Part print with two shaded views. Sizes in mm from the minimum x, y, z corner. Give positions to 0.01 mm unless a question says otherwise; leave off trailing zeros. Order: outer loops, then holes, each group sorted by start corner. A loop starts at its lowest first (then second) coordinate and runs counter-clockwise, first axis right, second up.
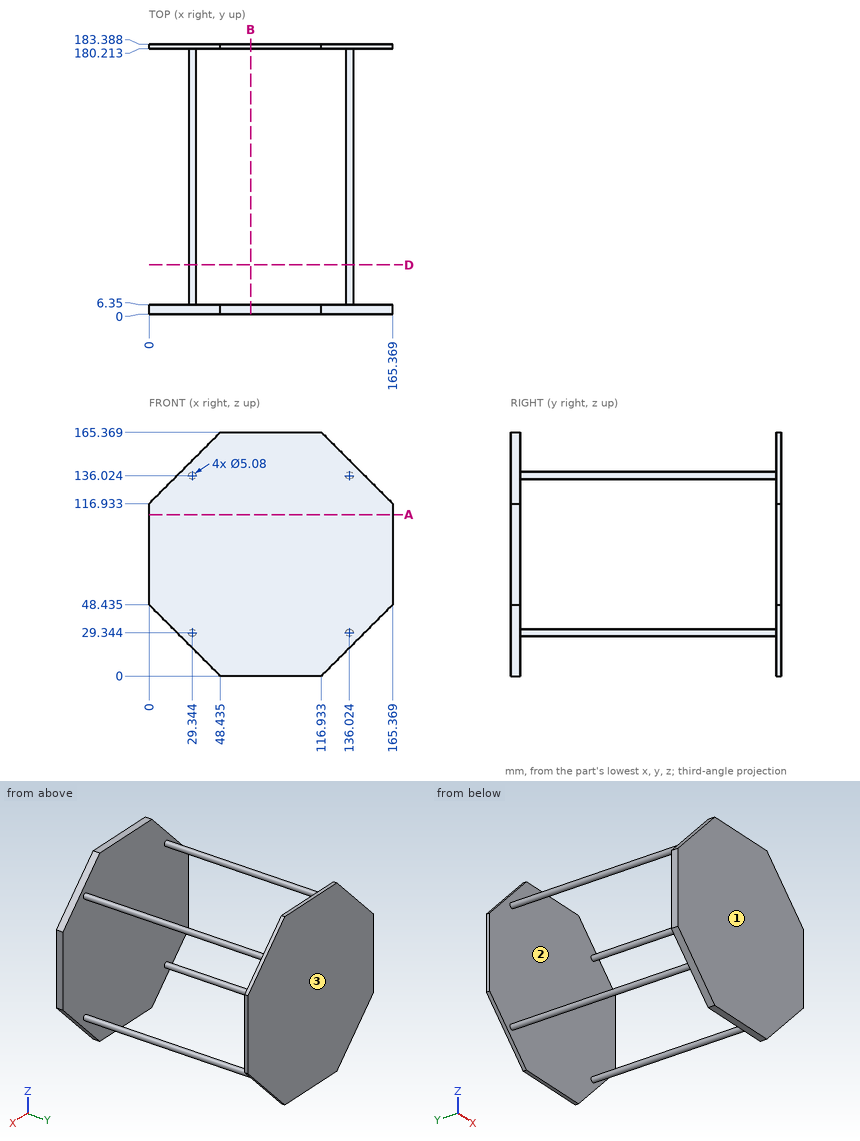
Item 1: Two-plate mould, pull along Y, no slides. Class the marked faces 1, 2 and 3: released by +Y, released by -Y, zero draft, split by the parting line, or undercut.
Item 2: Drop flat-ended pins along their axis: pin 1 Ø6 at (x, z) = (108.5, 73) entering from -Y; pin 2 Ø12 at (x, y) = (41.5, 66) entering from +Z; pin 3 Ø1.5 at (x, y) = (135, 35.5) entering from +Z. Give the stop position or say it passes through.
Item 3: Slice it at D-D (y = 33.5). Give the cut face in (x, z) (1 decimal).
Item 4: Wall check: L1, parallel to Y at x = 29.5, z = 94.5; L2, parallel to Z at x = 30, y = 133; L3, parallel to Z at x = 134.5, y = 98 (1 decimal). Give the ranges that are in metal, low to high.
Item 5: Slice it at A-A (z = 109.5). Give the cut face in (x, y).
Item 6: Slice it at B-B (x = 69). Give the cut face in (y, z).
A:
1. face 1: released by -Y
1. face 2: undercut
1. face 3: released by +Y
2. pin 1: stops at y = 0
2. pin 2: passes through
2. pin 3: stops at z = 138.55
3. outline: circle Ø5.1 at (29.3, 29.3); circle Ø5.1 at (29.3, 136); circle Ø5.1 at (136, 29.3); circle Ø5.1 at (136, 136)
4. L1: y = 0 to 6.35, 180.21 to 183.39
4. L2: z = 26.89 to 31.8, 133.57 to 138.48
4. L3: z = 27.3 to 31.4, 134 to 138.1
5. outline: (0, 0) - (165.37, 0) - (165.37, 6.35) - (0, 6.35) - close; (0, 180.21) - (165.37, 180.21) - (165.37, 183.39) - (0, 183.39) - close
6. outline: (0, 0) - (6.35, 0) - (6.35, 165.37) - (0, 165.37) - close; (180.21, 0) - (183.39, 0) - (183.39, 165.37) - (180.21, 165.37) - close
